CAD build for the part. Positions are in the model's coordinates, mm. A direction names the side the tool comes from. Round coordinates to 2 decimals unless told otherwise and drop trailing zeros. Loops run counter-clockwise (first coordinate to the right, second up) from the corner with the lowest first, then second, coordinate; pieces in that order, holes last.
from build123d import *

# Parameters (mm, degrees)
SKETCH1_R           = 13.5
SKETCH1_R_2         = 12.5
BOSS_EXTRUDE1_DEPTH = 10
CUT_EXTRUDE1_DEPTH  = 4


with BuildPart() as part:
    # Sketch1 → Boss-Extrude1 (new body)
    with BuildSketch(Plane(origin=(0, 0, 0), x_dir=(1, 0, 0), z_dir=(0, 1, 0))):
        with Locations(Location((0, 0, 0), (0, 0, 270))):
            Circle(SKETCH1_R)
        with Locations(Location((0, 0, 0), (0, 0, 270))):
            Circle(SKETCH1_R_2, mode=Mode.SUBTRACT)
    extrude(amount=BOSS_EXTRUDE1_DEPTH)

    # Sketch2 → Cut-Extrude1 (cut)
    with BuildSketch(Plane(origin=(0, 10, 0), x_dir=(1, 0, 0), z_dir=(0, 1, 0))):
        Polygon((-45.033320997, 13.5), (0, -12.5), (45.033320997, 13.5), align=None)
    extrude(amount=-CUT_EXTRUDE1_DEPTH, mode=Mode.SUBTRACT)


solid = part.part
Item 1: Cut at C-C (y = 4). List the corners of the cut face in (x, z).
Verdict:
outline: circle Ø27 at (0, 0); hole circle Ø25 at (0, 0)
Item 2: Flat gauge pins, fed straight in: P1, Ø10, axis at x = -0.5, z = -8, coming from the +Y side; P2, Ø3, axis at x = -5.5, y = 4, coming from the -Z side; P3, Ø1, axis at y = 3, z = -3.5, coming from the -X side. Where does each tip first touch, or does it go through?
Verdict:
P1: stops at y = 6
P2: stops at z = -12.89
P3: stops at x = -13.16
Item 3: Mould opens along X. For faces 1 (the flat face through (-11.62, 8.03, 5.79)), 2 (the flat face through (0, 10, 13)), 3 (the cylindrical face through (-5.17, 3.82, 12.47)) say: released by +X, released by -X, zero draft, split by the parting line, or undercut.
Verdict:
face 1: undercut
face 2: zero draft
face 3: split by the parting line
Item 4: Wall check: L1, parallel to X at y = 3, z = 0; L2, parallel to X at y = 5.5, z = 9; L3, parallel to Z at x = 0, y = 6.5. Give the ranges that are in metal, low to high.
Verdict:
L1: x = -13.5 to -12.5, 12.5 to 13.5
L2: x = -10.06 to -8.67, 8.67 to 10.06
L3: z = 12.5 to 13.5
Item 5: 3-axis set-ups, long thin cutter, end or side, ignore diameter. For faces 4 (the flat face through (11.601, 8.028, 5.802)), 5 (the cylindrical face through (3.755, 3.819, 11.923)): which of +Z, -Z, +X, -X, +Y, -Y reach the whole face in a straight line?
Verdict:
face 4: -Z, +Y
face 5: +Y, -Y
Item 6: Cut at D-D (y = 9). List the corners of the cut face in (x, z), plus the area to 3 significant figures.
Verdict:
outline: (-12.4, 5.34) - (-10.83, 6.25) arc R12.5 cw to (10.83, 6.25) - (12.4, 5.34) arc R13.5 ccw to start
area: 28.8 mm2
Item 7: Cut at A-A (x = 0). List the corners of the cut face in (y, z).
Verdict:
outline: (0, -13.5) - (6, -13.5) - (6, -12.5) - (0, -12.5) - close; (0, 12.5) - (10, 12.5) - (10, 13.5) - (0, 13.5) - close
Item 8: Cut at B-B (z = -7.5). List the corners of the cut face in (x, y), plus the area to 3 significant figures.
Verdict:
outline: (-11.22, 0) - (-10, 0) - (-10, 6) - (-11.22, 6) - close; (10, 0) - (11.22, 0) - (11.22, 6) - (10, 6) - close
area: 14.7 mm2
